```python
from build123d import *

# Parameters (mm, degrees)
SKETCH2_W               = 58.7502
SKETCH2_H               = 8.636
BOSS_EXTRUDE1_DEPTH     = 4.699
CUT_EXTRUDE1_DEPTH      = 1
CUT_EXTRUDE1_DEPTH_BACK = 3.175


with BuildPart() as part:
    # Sketch2 → Boss-Extrude1 (new body)
    with BuildSketch(Plane(origin=(0, 0, 0), x_dir=(1, 0, 0), z_dir=(0, 1, 0))):
        with Locations((-0.882327606, -0.31486737)):
            Rectangle(SKETCH2_W, SKETCH2_H)
    extrude(amount=BOSS_EXTRUDE1_DEPTH)

    # Sketch5 → Cut-Extrude1 (cut, two sides)
    with BuildSketch(Plane.XY.offset(4.63286737)) as cut_extrude1_sk:
        Polygon((-0.882327606, 0), (-2.863527606, 0), (-2.863527606, 4.699), (1.098872394, 4.699), (1.098872394, 0), align=None)
    extrude(amount=CUT_EXTRUDE1_DEPTH, mode=Mode.SUBTRACT)
    extrude(cut_extrude1_sk.sketch, amount=-CUT_EXTRUDE1_DEPTH_BACK, mode=Mode.SUBTRACT)


solid = part.part
```
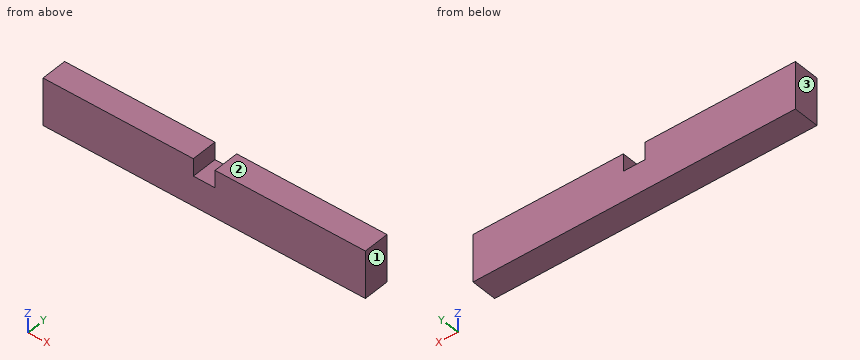
Work out the finished part from the listing and answer in its coordinate system (mm). Face numbers are marked on the shaded views. Give positions to 0.01 mm unless a question says otherwise; leave off trailing zeros. Write each loop counter-clockwise with the first axis right and the second up, starting at its lowest first coordinate (ties: lowest second). Pieces come first, ordered by that corner, then holes. Notation, with made-up numbers: (30.25, 6.5) - (73.25, 6.5) arc R30 ccw to (73.25, 40.5) - close; hole circle Ø5 at (65.5, -26). An arc over 180 degrees is marked (long way). Use one line per item in the form item = value.
1. Consider L1, parallel to X at y = 3.1, z = 1.75. Determine where the line is inside the solid, lowest interval first.
Filled in:
L1 = -30.26 to -2.86, 1.1 to 28.49
2. A cutting plane is placed at A-A (y = 3.1). Write down the section's boundary in (x, z).
Filled in:
outline = (-30.26, -4) - (28.49, -4) - (28.49, 4.63) - (1.1, 4.63) - (1.1, 1.46) - (-2.86, 1.46) - (-2.86, 4.63) - (-30.26, 4.63) - close
3. Determine the mould class of the marked faces 1, 2 and 3 for opening direction X: released by +X, released by -X, zero draft, split by the parting line, or undercut.
Filled in:
face_1 = released by +X
face_2 = zero draft
face_3 = released by -X
4. A cutting plane is placed at C-C (x = -0.5). Write down the section's boundary in (y, z).
Filled in:
outline = (0, -4) - (4.7, -4) - (4.7, 1.46) - (0, 1.46) - close
5. A cutting plane is placed at B-B (z = 2.75). Write down the section's boundary in (x, y), and give its area (3 significant figures).
Filled in:
outline = (-30.26, 0) - (-2.86, 0) - (-2.86, 4.7) - (-30.26, 4.7) - close; (1.1, 0) - (28.49, 0) - (28.49, 4.7) - (1.1, 4.7) - close
area = 257 mm^2
6. This flat-tipped pin is pushed along its axis until it touches: pin 1 Ø1.2 at (x, y) = (-1, 2) entering from +Z. Where does it stop, or does it pass through?
Filled in:
pin_1 = 1.46
